```python
from build123d import *

# Parameters (mm, degrees)
F0_W     = 82.55
F0_H     = 19.05
F1_DEPTH = 25.4
F3_DEPTH = 25.4
F4_R     = 9.525
F5_DEPTH = 25.4
F6_R     = 2.38125
F7_DEPTH = 25.4
F9_D     = 5.4102


with BuildPart() as f1:
    # F0 (on Front) → F1 (new body)
    with BuildSketch(Plane.XZ):
        with Locations((41.275, -9.525)):
            Rectangle(F0_W, F0_H)
    extrude(amount=F1_DEPTH)

    # F2 (on face) → F3 (cut)
    with BuildSketch(Plane.XY):
        with BuildLine():
            Line((26.3469211429, -5.969), (13.6469211429, -5.969))
            ThreePointArc((13.6469211429, -5.969), (6.9159211429, -12.7), (13.6469211429, -19.431))
            Line((13.6469211429, -19.431), (26.3469211429, -19.431))
            ThreePointArc((26.3469211429, -19.431), (33.0779211429, -12.7), (26.3469211429, -5.969))
        make_face()
    extrude(amount=-F3_DEPTH, mode=Mode.SUBTRACT)

    # F4 (on face) → F5 (cut)
    with BuildSketch(Plane.XZ.offset(25.4)):
        with Locations((16.764, 4.7625)):
            Circle(F4_R)
    extrude(amount=-F5_DEPTH, mode=Mode.SUBTRACT)

    # F6 (on face) → F7 (cut)
    with BuildSketch(Plane.XZ.offset(25.4)):
        with Locations((4.064, -20.16125)):
            Circle(F6_R)
    extrude(amount=-F7_DEPTH, mode=Mode.SUBTRACT)

    # F9 (through all)
    with Locations(Plane.XY):
        with Locations((76.835, -12.7)):
            Hole(F9_D / 2)


solid = f1.part
```
The listing builds one solid part. Answer for the finished solid, in the listing's coordinates (mm). A direction names the side the tool comes from. Give positions to 0.01 mm unless a question says otherwise; leave off trailing zeros. Write each loop counter-clockwise with the first axis right and the second up, starting at its lowest first coordinate (ties: lowest second). Pieces come first, ordered by that corner, then holes. Notation, with made-up numbers: (67, 20.5) - (113, 20.5) arc R25 cw to (113, 58.5) - close; hole circle Ø3 at (54.5, 7). An arc over 180 degrees is marked (long way). Use one line per item in the form item = value. Start each with the question number.
1) Consider line 1 along Y through (x, z) = (23.5, -4.5); line 2 along X through (y, z) = (-13.25, -1.75); line 3 along X through (y, z) = (-6.75, -5). Determine where each line is inside the solid, lowest interval first. Write a range as from..to.
2) Find section A-A on y = -12.7. Determine the outline of the cut face in (x, z).
3) The mould has two halves that part along Y. Classify faces 3 (the face through (4, -13, 0)), 4 (the face through (20, -19.431, -12)), 5 (the face through (41, 0, -9)): pulls with the +Y half, pulls with the -Y half, needs draft (parallel to the pull), parting line crosses it, or undercut.
4) A flat-ended cylindrical pin translates along its axis: pin 1 Ø4 at (x, y) = (27.5, -9) entering from +Z. Find the tip coordinate at first contact, or state that the pin passes through.
5) Find section C-C on z = -9. Determine the outline of the cut face in (x, y) (3 decimals).
6) Find section B-B on z = -1.75. Determine the outline of the cut face in (x, y) (3 decimals), plus the area to 3 significant figures.
7) A tool of negligible diameter and unlimited length cuts with its end or side. For faces 1 (the face through (1, -13, -19.05)), 2 (the face through (20, -5.969, -12)), from which of +Z, -Z, +X, -X, +Y, -Y can it reach the whole face along a straight path? Write none if from no direction.
Geometry results:
q1.line_1 = -25.4..-19.43, -5.97..0
q1.line_2 = 0..6.94, 33.06..74.19, 79.48..82.55
q1.line_3 = 0..10.5, 29.49..82.55
q2.outline = (0, -19.05) - (1.96, -19.05) arc R2.38 cw to (6.17, -19.05) - (6.92, -19.05) - (6.92, 0) - (0, 0) - close; (33.08, -19.05) - (74.13, -19.05) - (74.13, 0) - (33.08, 0) - close; (79.54, -19.05) - (82.55, -19.05) - (82.55, 0) - (79.54, 0) - close
q3.face_3 = needs draft
q3.face_4 = undercut
q3.face_5 = pulls with the +Y half
q4.pin_1 = through
q5.outline = (0, -25.4) - (82.55, -25.4) - (82.55, 0) - (0, 0) - close; hole (13.647, -19.431) - (26.347, -19.431) arc R6.731 ccw to (26.347, -5.969) - (13.647, -5.969) arc R6.731 ccw to start; hole circle Ø5.41 at (76.835, -12.7)
q6.outline = (0, -25.4) - (9.813, -25.4) - (9.813, -18.233) arc R6.731 cw to (9.813, -7.167) - (9.813, 0) - (0, 0) - close; (23.715, -25.4) - (82.55, -25.4) - (82.55, 0) - (23.715, 0) - (23.715, -5.969) - (26.347, -5.969) arc R6.731 cw to (26.347, -19.431) - (23.715, -19.431) - close; hole circle Ø5.41 at (76.835, -12.7)
q6.area = 1,590 mm2
q7.face_1 = -Z, +X, -X, +Y, -Y
q7.face_2 = +Z, -Z
